Read the model definition and answer for the solid it produces. Units are mm, in the model's axes. Face numbers are marked on the shaded views. A direction names the side the tool comes from. Round coordinates to 2 decimals unless told otherwise and drop trailing zeros. Write each loop counter-clockwise with the first axis right and the second up, starting at its lowest first coordinate (ties: lowest second). Pieces come first, ordered by that corner, then holes. Notation, with made-up numbers: (-12, 4.25) -> (22, 4.25) arc R19 ccw to (22, 36.25) -> close; hole circle Ø8 at (7.5, -21). An arc over 180 degrees is marked (long way). Return JSON: item names as keys, results as strings.
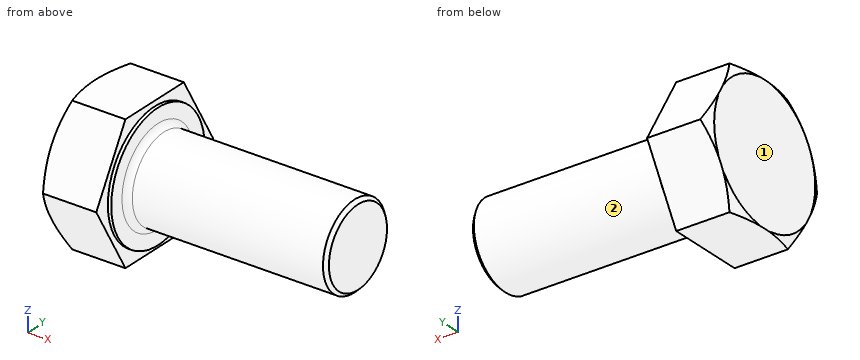
from build123d import *

# Parameters (mm, degrees)
ESTRUSIONE_ESTRUSIONE1_DEPTH = 3.5
SMUSSO1_SIZE                 = 0.2
RACCORDO1_R                  = 0.35


with BuildPart() as part:
    # Schizzo1 → Rivoluzione1 (revolve)
    with BuildSketch(Plane.XY):
        Polygon((0.2, 2.5), (12, 2.5), (12, 0), (0, 0), (0, 3.7), (0.2, 3.7), align=None)
    revolve(axis=Axis((12, 0, 0), (-1, 0, 0)))

    # Schizzo2 → Estrusione-Estrusione1 (add)
    with BuildSketch(Plane.ZY):
        Polygon((0, -4.618802154), (4, -2.309401077), (4, 2.309401077), (0, 4.618802154), (-4, 2.309401077), (-4, -2.309401077), align=None)
    extrude(amount=ESTRUSIONE_ESTRUSIONE1_DEPTH)

    # Schizzo3 → Taglia-Rivoluzione3 (revolve, cut)
    with BuildSketch(Plane.XY):
        Polygon((-3.5, 4), (-3.14273441, 4.618802154), (-3.5, 4.618802154), align=None)
    revolve(axis=Axis((0.2, 0, 0), (1, 0, 0)), mode=Mode.SUBTRACT)

    # Smusso1
    smusso1_edges = [part.edges().sort_by_distance(p)[0] for p in [
        (12, -2.5, 0),
    ]]
    chamfer(smusso1_edges, length=SMUSSO1_SIZE)

    # Raccordo1
    raccordo1_edges = [part.edges().sort_by_distance(p)[0] for p in [
        (0.2, -2.5, 0),
    ]]
    fillet(raccordo1_edges, radius=RACCORDO1_R)


solid = part.part
Item 1: Flat-ended cylindrical pins translate along their axes: pin 1 (2 mm diameter, centred on x = 2.5, y = 2.5, fed in from -Z); pin 2 (4 mm diameter, centred on x = 3, y = -2.5, fed in from +Z); pin 3 (2 mm diameter, centred on x = 8, z = -1.5, fed in from -Y). Find the tip coordinate at first contact, or state that the pin passes through.
Worked answers:
{"pin 1": "stops at z = -2", "pin 2": "stops at z = 2.45", "pin 3": "stops at y = -2.45"}
Item 2: A tool of negligible diameter and unlimited length cuts with its end or side. For the marked faces 1 and 2, from which of +Z, -Z, +X, -X, +Y, -Y can it reach the whole face along a straight path? Write none if from no direction.
Worked answers:
{"face 1": "+Z, -Z, -X, +Y, -Y", "face 2": "+X"}
Item 3: Section A-A (x = 8.25) is taken. Give the vertices of the cut face in (y, z).
Worked answers:
{"outline": "circle Ø5 at (0, 0)"}
Item 4: Straight lines are drawn through the part: L1, parallel to X at y = -2.75, z = -3; L2, parallel to Y at x = 11.75, z = 0; L3, parallel to X at y = -1, z = 3.5. For each, find the intervals that lie inside material, in ascending order. Write a range as [from, to].
Worked answers:
{"L1": "x = [-3.46, 0]", "L2": "y = [-2.5, 2.5]", "L3": "x = [-3.5, 0.2]"}
